```python
from build123d import *

# Parameters (mm, degrees)
SKETCH_1_W      = 120
SKETCH_1_H      = 40
SKETCH_1_R      = 2.25
EXTRUDE_1_DEPTH = 5
FILLET_1_R      = 2.5
FILLET_2_R      = 1


with BuildPart() as part:
    # 草图1 → 凸台-拉伸1 (new body)
    with BuildSketch(Plane.XY):
        Rectangle(SKETCH_1_W, SKETCH_1_H)
        with Locations((-56, -16)):
            Circle(SKETCH_1_R, mode=Mode.SUBTRACT)
        with Locations((-56, -8)):
            Circle(SKETCH_1_R, mode=Mode.SUBTRACT)
        with Locations((-56, 0)):
            Circle(SKETCH_1_R, mode=Mode.SUBTRACT)
        with Locations((-56, 8)):
            Circle(SKETCH_1_R, mode=Mode.SUBTRACT)
        with Locations((-56, 16)):
            Circle(SKETCH_1_R, mode=Mode.SUBTRACT)
        with Locations((56, 16)):
            Circle(SKETCH_1_R, mode=Mode.SUBTRACT)
        with Locations((56, 8)):
            Circle(SKETCH_1_R, mode=Mode.SUBTRACT)
        with Locations((56, 0)):
            Circle(SKETCH_1_R, mode=Mode.SUBTRACT)
        with Locations((56, -16)):
            Circle(SKETCH_1_R, mode=Mode.SUBTRACT)
        with Locations((56, -8)):
            Circle(SKETCH_1_R, mode=Mode.SUBTRACT)
        with Locations((-48, 16)):
            Circle(SKETCH_1_R, mode=Mode.SUBTRACT)
        with Locations((-48, 8)):
            Circle(SKETCH_1_R, mode=Mode.SUBTRACT)
        with Locations((-40, 16)):
            Circle(SKETCH_1_R, mode=Mode.SUBTRACT)
        with Locations((-40, 8)):
            Circle(SKETCH_1_R, mode=Mode.SUBTRACT)
        with Locations((-32, 16)):
            Circle(SKETCH_1_R, mode=Mode.SUBTRACT)
        with Locations((-32, 8)):
            Circle(SKETCH_1_R, mode=Mode.SUBTRACT)
        with Locations((-24, 16)):
            Circle(SKETCH_1_R, mode=Mode.SUBTRACT)
        with Locations((-24, 8)):
            Circle(SKETCH_1_R, mode=Mode.SUBTRACT)
        with Locations((-16, 16)):
            Circle(SKETCH_1_R, mode=Mode.SUBTRACT)
        with Locations((-16, 8)):
            Circle(SKETCH_1_R, mode=Mode.SUBTRACT)
        with Locations((-8, 16)):
            Circle(SKETCH_1_R, mode=Mode.SUBTRACT)
        with Locations((-8, 8)):
            Circle(SKETCH_1_R, mode=Mode.SUBTRACT)
        with Locations((0, 16)):
            Circle(SKETCH_1_R, mode=Mode.SUBTRACT)
        with Locations((0, 8)):
            Circle(SKETCH_1_R, mode=Mode.SUBTRACT)
        with Locations((8, 16)):
            Circle(SKETCH_1_R, mode=Mode.SUBTRACT)
        with Locations((8, 8)):
            Circle(SKETCH_1_R, mode=Mode.SUBTRACT)
        with Locations((16, 16)):
            Circle(SKETCH_1_R, mode=Mode.SUBTRACT)
        with Locations((16, 8)):
            Circle(SKETCH_1_R, mode=Mode.SUBTRACT)
        with Locations((24, 16)):
            Circle(SKETCH_1_R, mode=Mode.SUBTRACT)
        with Locations((24, 8)):
            Circle(SKETCH_1_R, mode=Mode.SUBTRACT)
        with Locations((32, 16)):
            Circle(SKETCH_1_R, mode=Mode.SUBTRACT)
        with Locations((32, 8)):
            Circle(SKETCH_1_R, mode=Mode.SUBTRACT)
        with Locations((40, 16)):
            Circle(SKETCH_1_R, mode=Mode.SUBTRACT)
        with Locations((40, 8)):
            Circle(SKETCH_1_R, mode=Mode.SUBTRACT)
        with Locations((48, 16)):
            Circle(SKETCH_1_R, mode=Mode.SUBTRACT)
        with Locations((48, 8)):
            Circle(SKETCH_1_R, mode=Mode.SUBTRACT)
        with BuildLine():
            Line((20, -8), (-20, -8))
            ThreePointArc((-20, -8), (-22, -10), (-20, -12))
            Line((-20, -12), (20, -12))
            ThreePointArc((20, -12), (22, -10), (20, -8))
        make_face(mode=Mode.SUBTRACT)
    extrude(amount=EXTRUDE_1_DEPTH)

    # 圆角1
    fillet_1_edges = [part.edges().sort_by_distance(p)[0] for p in [
        (60, -20, 2.5),
        (-60, -20, 2.5),
        (-60, 20, 2.5),
        (60, 20, 2.5),
    ]]
    fillet(fillet_1_edges, radius=FILLET_1_R)

    # 圆角2
    fillet_2_edges = [part.edges().sort_by_distance(p)[0] for p in [
        (0, -8, 5),
        (22, -10, 5),
        (0, -12, 5),
        (-22, -10, 5),
    ]]
    fillet(fillet_2_edges, radius=FILLET_2_R)


solid = part.part
```
Can you work these out from the model? Positions are in its coordinate system, mm. Give positions to 0.01 mm unless a question says otherwise; leave off trailing zeros. Loops run counter-clockwise (first coordinate to the right, second up) from the corner with the lowest first, then second, coordinate; pieces in that order, holes last. Notation, with made-up numbers: M 47.5,81 L 75.5,81 A26 ccw 75.5,119 Z; hole C 52.25,-34 d3. An arc over 180 degrees is marked long. One line per question, with ' | ' between items. Start each with the question number.
Q1. If we section it at B-B (x = 40): Please give me the cut outline in (y, z).
Q2. If we mould it in two halves opening along X, with no side actions, what happens to faces 1 (the cylindrical face through (59.248, 19.287, 2.535)), 2 (the flat face through (-1, 0, 0)), 3 (the cylindrical face through (-30.79, 9.897, 2.465))? For each: +X half, -X half, draft (parallel to the pull), parting line (faces both ways), or undercut.
Q3. If I drill on line 1 (Y direction, x = -56, z = 2.25); line 2 (Y direction, x = -48, z = 3.65); line 3 (Y direction, x = 8, z = 2), over which ranges is the centre line in solid material (lowest first)? Write a range as from..to.
Q4. If we section it at C-C (y = -16): Please give me the cut outline in (x, z).
Q5. If we section it at A-A (x = 56): Please give me the cut outline in (y, z), plus the area to 3 significant figures.
Q6. If we section it at D-D (x = 16): Please give me the cut outline in (y, z).
Computed:
1) outline: M -20,0 L 5.75,0 L 5.75,5 L -20,5 Z; M 10.25,0 L 13.75,0 L 13.75,5 L 10.25,5 Z; M 18.25,0 L 20,0 L 20,5 L 18.25,5 Z
2) face 1: +X half | face 2: draft | face 3: undercut
3) line 1: y = -20..-18.25, -13.75..-10.25, -5.75..-2.25, 2.25..5.75, 10.25..13.75, 18.25..20 | line 2: y = -20..5.75, 10.25..13.75, 18.25..20 | line 3: y = -20..-12, -8..5.75, 10.25..13.75, 18.25..20
4) outline: M -60,0 L -58.25,0 L -58.25,5 L -60,5 Z; M -53.75,0 L 53.75,0 L 53.75,5 L -53.75,5 Z; M 58.25,0 L 60,0 L 60,5 L 58.25,5 Z
5) outline: M -20,0 L -18.25,0 L -18.25,5 L -20,5 Z; M -13.75,0 L -10.25,0 L -10.25,5 L -13.75,5 Z; M -5.75,0 L -2.25,0 L -2.25,5 L -5.75,5 Z; M 2.25,0 L 5.75,0 L 5.75,5 L 2.25,5 Z; M 10.25,0 L 13.75,0 L 13.75,5 L 10.25,5 Z; M 18.25,0 L 20,0 L 20,5 L 18.25,5 Z | area: 87.5 mm²
6) outline: M -20,0 L -12,0 L -12,4 A1 ccw -13,5 L -20,5 Z; M -8,0 L 5.75,0 L 5.75,5 L -7,5 A1 ccw -8,4 Z; M 10.25,0 L 13.75,0 L 13.75,5 L 10.25,5 Z; M 18.25,0 L 20,0 L 20,5 L 18.25,5 Z
